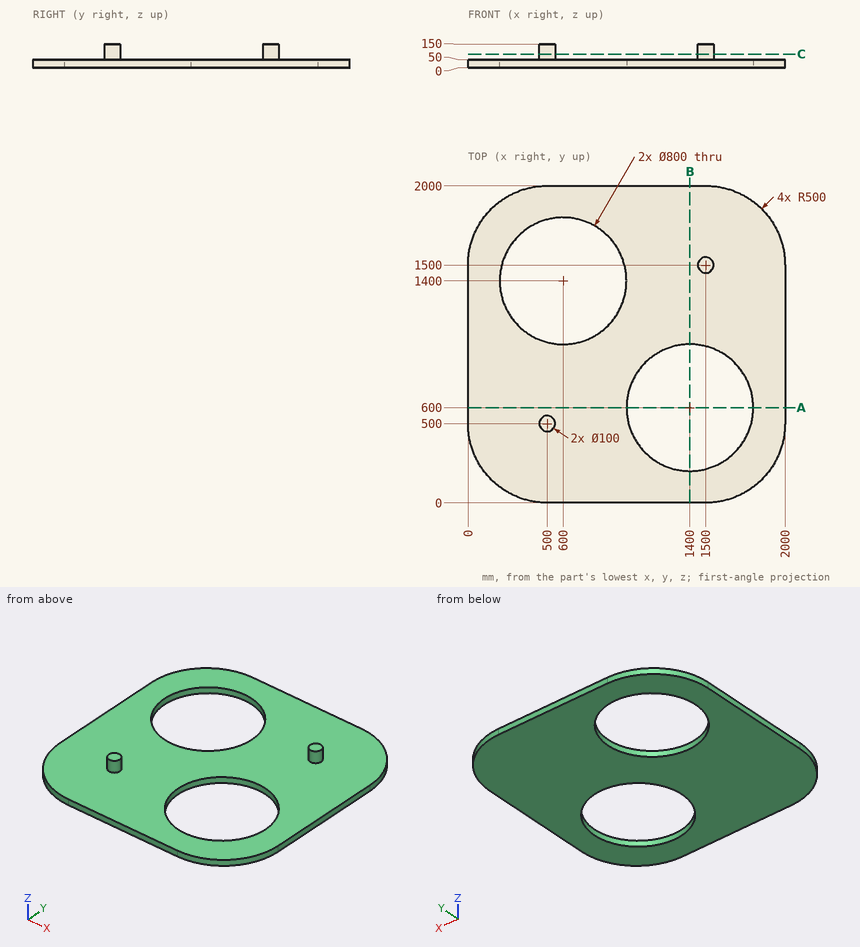
Input: dimensioned drawing with shaded views. Units: mm. Origin: part minimum x, y, z. Give positions to 0.01 mm unless a question says otherwise; leave off trailing zeros. Order: outer loops, then holes, each group sorted by start corner. A loop starts at its lowest first (then second) coordinate and runs counter-clockwise, first axis right, second up.
(1) Section query C-C (z = 86.5). Return the cut outline in (x, y), plus the area to 3 significant figures.
(2) Section query A-A (y = 600). Return the cut outline in (x, z).
(3) Section query B-B (x = 1400). Return the cut outline in (y, z).
(4) Contact query for a flat-ended pin moving along its axis: P1, Ø2, axis at x = 1103.5, y = 1181, coming from the +Z side. Output: stop coordinate, or through.
(5) Material intervals for line 1 along Y through (x, z) = (600, 22.5); line 2 along Y through (x, z) = (1400, 15); line 3 along Z through (x, y) = (1648.5, 1590), sorted ascending.
Outcome:
1. outline: circle Ø100 at (500, 500); circle Ø100 at (1500, 1500)
1. area: 15,700 mm2
2. outline: (0, 0) - (1000, 0) - (1000, 50) - (0, 50) - close; (1800, 0) - (2000, 0) - (2000, 50) - (1800, 50) - close
3. outline: (0, 0) - (200, 0) - (200, 50) - (0, 50) - close; (1000, 0) - (2000, 0) - (2000, 50) - (1000, 50) - close
4. P1: stops at z = 50
5. line 1: y = 0 to 1000, 1800 to 2000
5. line 2: y = 0 to 200, 1000 to 2000
5. line 3: z = 0 to 50
